Verification items for the finished model (mm, model axes). Face numbers are marked on the shaded views. A direction names the side the tool comes from. Give positions to 0.01 mm unless a question says otherwise; leave off trailing zeros. Write each loop counter-clockwise with the first axis right and the second up, starting at its lowest first coordinate (ties: lowest second). Pieces come first, ordered by that corner, then holes. Notation, with made-up numbers: (-1.75, -30) -> (15.25, -30) arc R10 ccw to (15.25, -17) -> close; hole circle Ø9 at (65.5, 69.5). An arc over 180 degrees is marked (long way). Use CSV: the item, a comma, the result in double quotes. Start each with the question number.
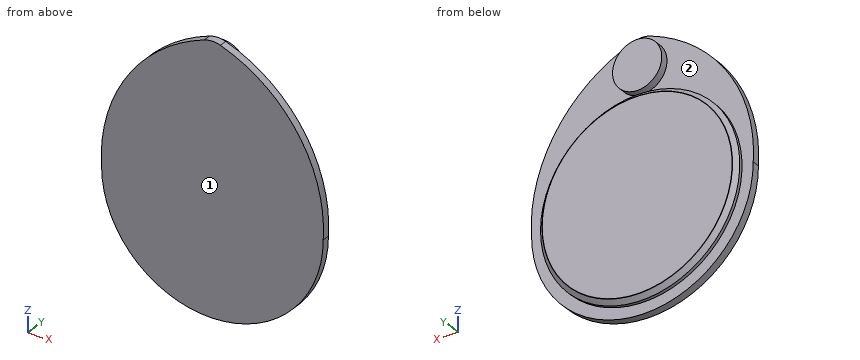
```python
from build123d import *

# Parameters (mm, degrees)
SKETCH1_R           = 44.5
BOSS_EXTRUDE1_DEPTH = 3.5
CHAMFER1_SIZE       = 2
SKETCH2_R           = 49.5
BOSS_EXTRUDE2_DEPTH = 3.5
BOSS_EXTRUDE3_DEPTH = 3.5
SKETCH7_R           = 10.991686932
BOSS_EXTRUDE4_DEPTH = 3.5
FILLET1_R           = 11
FILLET2_R           = 0.25


with BuildPart() as part:
    # Sketch1 → Boss-Extrude1 (new body)
    with BuildSketch(Plane(origin=(0, 0, 0), x_dir=(1, 0, 0), z_dir=(0, 1, 0))):
        Circle(SKETCH1_R)
    extrude(amount=BOSS_EXTRUDE1_DEPTH)

    # Chamfer1
    chamfer1_edges = [part.edges().sort_by_distance(p)[0] for p in [
        (-44.5, 3.5, 0),
    ]]
    chamfer(chamfer1_edges, length=CHAMFER1_SIZE)

    # Sketch2 → Boss-Extrude2 (add)
    with BuildSketch(Plane.XZ):
        Circle(SKETCH2_R)
    extrude(amount=BOSS_EXTRUDE2_DEPTH)

    # Sketch3 → Boss-Extrude3 (add)
    with BuildSketch(Plane(origin=(0, 0, 0), x_dir=(1, 0, 0), z_dir=(0, 1, 0))):
        with BuildLine():
            ThreePointArc((49.5, 0), (37.061785537, -43.706191201), (0, -70))
            ThreePointArc((0, -70), (-37.061785537, -43.706191201), (-49.5, 0))
            ThreePointArc((-49.5, 0), (0, -49.5), (49.5, 0))
        make_face()
    extrude(amount=-BOSS_EXTRUDE3_DEPTH)

    # Sketch7 → Boss-Extrude4 (add)
    with BuildSketch(Plane(origin=(0, 0, 0), x_dir=(1, 0, 0), z_dir=(0, 1, 0))):
        with Locations((0, -55.892027532)):
            Circle(SKETCH7_R)
    extrude(amount=BOSS_EXTRUDE4_DEPTH)

    # Fillet1
    fillet1_edges = [part.edges().sort_by_distance(p)[0] for p in [
        (0, -1.75, 70),
    ]]
    fillet(fillet1_edges, radius=FILLET1_R)

    # Fillet2
    fillet2_edges = [part.edges().sort_by_distance(p)[0] for p in [
        (-42.5, 3.5, 0),
    ]]
    fillet(fillet2_edges, radius=FILLET2_R)


solid = part.part
```
(1) Go/stop test with flat-tipped pins: pin 1 (1 mm diameter, centred on y = -2, z = -11.5, fed in from +X); pin 2 (1 mm diameter, centred on x = 37.5, y = -1.5, fed in from -Z). Record where each tip stops, or that it passes through.
(2) Thickness scan on line 1 (Y direction, x = 17, z = 53); line 2 (X direction, y = -2.5, z = -25.5); line 3 (Z direction, x = 4.5, y = 2.25). Record the ranges inside material, lowest first. Write a range as from..to.
(3) Set-up check for the marked faces 1 and 2: record each of +Z, -Z, +X, -X, +Y, -Y from which the full face is reachable in a straight line by a thin tool's end or side.
(4) Section check A-A on z = 50. Record the cut outline in (x, y).
Data:
1,pin 1,"stops at x = 48.26"
1,pin 2,"stops at z = -32.88"
2,line 1,"y = -3.5..0"
2,line 2,"x = -42.43..42.43"
2,line 3,"z = -43.52..43.52, 45.86..65.92"
3,face 1,"+Z, -Z, +X, -X, -Y"
3,face 2,"+Y"
4,outline,"(-32.03, -3.5) -> (32.03, -3.5) -> (32.03, 0) -> (9.28, 0) -> (9.28, 3.5) -> (-9.28, 3.5) -> (-9.28, 0) -> (-32.03, 0) -> close"
